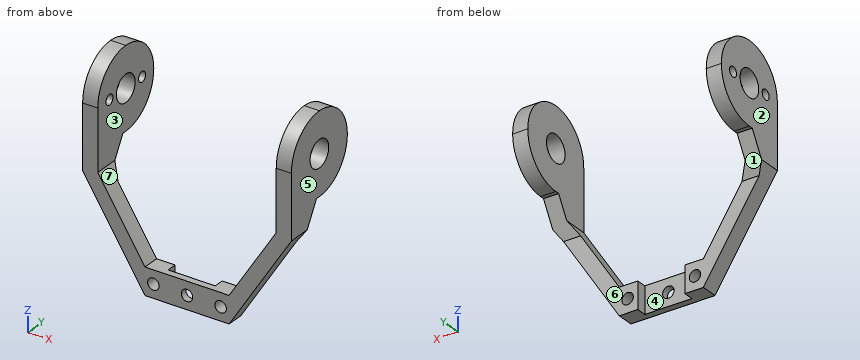
from build123d import *
from OCP.BRepFilletAPI import BRepFilletAPI_MakeChamfer

# Parameters (mm, degrees)
BOSS_EXTRUDE1_DEPTH     = 5
SKETCH2_W               = 4.5
SKETCH2_H               = 24
BOSS_EXTRUDE2_DEPTH     = 19
CUT_EXTRUDE1_REACH      = 59.853
SKETCH5_R               = 1.7
CUT_EXTRUDE2_REACH      = 73.673
SKETCH6_W               = 14
SKETCH6_H               = 3
CUT_EXTRUDE3_REACH      = 78.859
SKETCH7_R               = 1.5
CUT_EXTRUDE4_DEPTH      = 77.85863647
CUT_EXTRUDE4_DEPTH_BACK = 77.85863647
SKETCH8_R               = 4
FILLET1_R               = 12
CHAMFER2_SIZE           = 10
CHAMFER2_SIZE2          = 5.773502692
CUT_EXTRUDE5_REACH      = 59.853
SKETCH10_R              = 1.7


with BuildPart() as part:
    # Sketch1 → Boss-Extrude1 (new body)
    with BuildSketch(Plane(origin=(0, 0, 0), x_dir=(1, 0, 0), z_dir=(0, 1, 0))):
        Polygon((-31, 15.928571429), (-31, -15), (-26.5, -15), (-26.5, 15), (-12.5, 37), (12.5, 37), (26.5, 15), (26.5, -15), (31, -15), (31, 15.928571429), (12.5, 45), (-12.5, 45), align=None)
    extrude(amount=BOSS_EXTRUDE1_DEPTH)

    # Sketch2 → Boss-Extrude2 (add)
    with BuildSketch(Plane(origin=(0, 5, 0), x_dir=(1, 0, 0), z_dir=(0, 1, 0))):
        with Locations((-28.75, -3)):
            Rectangle(SKETCH2_W, SKETCH2_H)
        with Locations((28.75, -3)):
            Rectangle(SKETCH2_W, SKETCH2_H)
    extrude(amount=BOSS_EXTRUDE2_DEPTH)

    # Sketch5 → Cut-Extrude1 (cut, up to next)
    with BuildSketch(Plane(origin=(0, 5, 0), x_dir=(1, 0, 0), z_dir=(0, 1, 0)), mode=Mode.PRIVATE) as cut_extrude1_sk1:
        with Locations(Location((0, 41, 0), (0, 0, 270))):
            Circle(SKETCH5_R)
    cut_extrude1_tool1 = extrude(cut_extrude1_sk1.sketch, amount=-CUT_EXTRUDE1_REACH, mode=Mode.PRIVATE) & part.part
    add(cut_extrude1_tool1.solids().sort_by_distance((0, 5, -41))[0], mode=Mode.SUBTRACT)

    # Cut-Extrude2: up to this face of the body (flat: up to its plane)
    cut_extrude2_end = Plane(part.part.faces().sort_by_distance((0, 2.5, -37))[0])
    # Sketch6 → Cut-Extrude2 (cut, up to the picked face)
    with BuildSketch(Plane(origin=(0, 0, -45), x_dir=(-1, 0, 0), z_dir=(0, 0, -1)), mode=Mode.PRIVATE) as cut_extrude2_sk1:
        with Locations((0, 3.5)):
            Rectangle(SKETCH6_W, SKETCH6_H)
    cut_extrude2_tool1 = split(extrude(cut_extrude2_sk1.sketch, amount=-CUT_EXTRUDE2_REACH, mode=Mode.PRIVATE), bisect_by=cut_extrude2_end, keep=Keep.BOTH, mode=Mode.PRIVATE)
    add(cut_extrude2_tool1.solids().sort_by(Axis((0, 3.5, -45), (0, 0, 1)))[0], mode=Mode.SUBTRACT)

    # Sketch7 → Cut-Extrude3 (cut, up to next)
    with BuildSketch(Plane(origin=(-26.5, 0, 0), x_dir=(0, 0, -1), z_dir=(1, 0, 0)), mode=Mode.PRIVATE) as cut_extrude3_sk1:
        with Locations((-3, 19)):
            Circle(SKETCH7_R)
    cut_extrude3_tool1 = extrude(cut_extrude3_sk1.sketch, amount=-CUT_EXTRUDE3_REACH, mode=Mode.PRIVATE) & part.part
    # Sketch7 → Cut-Extrude3 (cut, up to next)
    with BuildSketch(Plane(origin=(-26.5, 0, 0), x_dir=(0, 0, -1), z_dir=(1, 0, 0)), mode=Mode.PRIVATE) as cut_extrude3_sk2:
        with Locations((-3, 5)):
            Circle(SKETCH7_R)
    cut_extrude3_tool2 = extrude(cut_extrude3_sk2.sketch, amount=-CUT_EXTRUDE3_REACH, mode=Mode.PRIVATE) & part.part
    add(cut_extrude3_tool1.solids().sort_by_distance((-26.5, 19, 3))[0], mode=Mode.SUBTRACT)
    add(cut_extrude3_tool2.solids().sort_by_distance((-26.5, 5, 3))[0], mode=Mode.SUBTRACT)

    # Sketch8 → Cut-Extrude4 (cut, two sides: drawn at the far end of the back side and taken through both)
    with BuildSketch(Plane(origin=(-26.5, 0, 0), x_dir=(0, 0, -1), z_dir=(1, 0, 0)).offset(-CUT_EXTRUDE4_DEPTH_BACK)):
        with Locations((-3, 12)):
            Circle(SKETCH8_R)
    extrude(amount=CUT_EXTRUDE4_DEPTH + CUT_EXTRUDE4_DEPTH_BACK, mode=Mode.SUBTRACT)

    # Fillet1
    fillet1_edges = [part.edges().sort_by_distance(p)[0] for p in [
        (28.75, 0, 15),
        (-28.75, 0, 15),
        (-28.75, 24, -9),
        (28.75, 24, -9),
        (28.75, 24, 15),
        (-28.75, 24, 15),
    ]]
    fillet(fillet1_edges, radius=FILLET1_R - 0.0001)  # a hair under: the kernel refuses the full size

    # Chamfer2: one chamfer whose edges measure the first distance from different faces: ONE call of the kernel's chamfer builder (chamfer() names one face for all edges)
    chamfer2_edges_1 = [part.edges().sort_by_distance(p)[0] for p in [
        (-28.75, 5, -9),
    ]]
    chamfer2_side_1 = [part.faces().sort_by_distance(p)[0] for p in [
        (-19.473621736, 5, -28.773341624),
    ]]
    chamfer2_edges_2 = [part.edges().sort_by_distance(p)[0] for p in [
        (28.75, 5, -9),
    ]]
    chamfer2_side_2 = [part.faces().sort_by_distance(p)[0] for p in [
        (19.473621736, 5, -28.773341624),
    ]]
    chamfer2 = BRepFilletAPI_MakeChamfer(part.part.solid().wrapped)
    for e in chamfer2_edges_1:
        chamfer2.Add(CHAMFER2_SIZE, CHAMFER2_SIZE2, e.wrapped, chamfer2_side_1[0].wrapped)  # the first distance lies on this face
    for e in chamfer2_edges_2:
        chamfer2.Add(CHAMFER2_SIZE, CHAMFER2_SIZE2, e.wrapped, chamfer2_side_2[0].wrapped)  # the first distance lies on this face
    add(Compound.cast(chamfer2.Shape()), mode=Mode.REPLACE)

    # Sketch10 → Cut-Extrude5 (cut, up to next)
    with BuildSketch(Plane(origin=(0, 5, 0), x_dir=(1, 0, 0), z_dir=(0, 1, 0)), mode=Mode.PRIVATE) as cut_extrude5_sk1:
        with Locations(Location((-10, 41, 0), (0, 0, 270))):
            Circle(SKETCH10_R)
    cut_extrude5_tool1 = extrude(cut_extrude5_sk1.sketch, amount=-CUT_EXTRUDE5_REACH, mode=Mode.PRIVATE) & part.part
    cut_extrude5 = cut_extrude5_tool1.solids().sort_by_distance((-10, 5, -41))[0]
    add(cut_extrude5, mode=Mode.SUBTRACT)

    # Mirror1: Cut-Extrude5 across plane
    add(cut_extrude5.mirror(Plane(origin=(0, 0, 0), x_dir=(0, 0, 1), z_dir=(1, 0, 0))), mode=Mode.SUBTRACT)


solid = part.part
Here's how the part is built. I have some questions about the finished solid (model axes, mm). Face numbers are marked on the shaded views. A direction names the side the tool comes from. Coordinates: 2 decimals unless noted, no trailing zeros. Order: outer loops, then holes, each group sorted by start corner. A loop starts at its lowest first (then second) coordinate and runs counter-clockwise, first axis right, second up.
Item 1: For P1, Ø5.5, axis at x = -10, z = -41, coming from the +Y side; P2, Ø12, axis at x = -18.5, z = 4.5, coming from the +Y side; P3, Ø1.5, axis at x = 3, y = 2.5, coming from the +Z side; P4, Ø0.9, axis at y = 4, z = -42.5, coming from the -X side, each with a flat end and sliding along its axis, tell me the tip position at first contact or that it passes through.
Result sheet:
P1: stops at y = 5
P2: passes through
P3: stops at z = -37
P4: stops at x = -14.38
Item 2: If we section it at C-C on y = 9.75: List the corners of the cut face in (x, z) for me, plus the area to 3 significant figures.
Result sheet:
outline: (-31, -10.77) - (-26.5, -10.77) - (-26.5, -0.31) - (-31, -0.31) - close; (-31, 6.31) - (-26.5, 6.31) - (-26.5, 14.79) - (-31, 14.79) - close; (26.5, -10.77) - (31, -10.77) - (31, -0.31) - (26.5, -0.31) - close; (26.5, 6.31) - (31, 6.31) - (31, 14.79) - (26.5, 14.79) - close
area: 171 mm2
Item 3: If we section it at A-A on x = 0: List the corners of the cut face in (y, z) for me, plus the area to 3 significant figures.
Result sheet:
outline: (0, -45) - (2, -45) - (2, -42.7) - (0, -42.7) - close; (0, -39.3) - (2, -39.3) - (2, -37) - (0, -37) - close
area: 9.20 mm2
Item 4: For the marked faces 5, 6 and 7, which set-ups out of +Z, -Z, +X, -X, +Y, -Y let a thin tool reach every point of the face, with its end or its side?
Result sheet:
face 5: +Z, -Z, +X, +Y, -Y
face 6: -Z, +X, -X, +Y
face 7: +Z, +Y, -Y
Item 5: I need wall thicknesses on line 1 (Y direction, x = -28.3, z = 3); line 2 (X direction, y = 13, z = -3.5); line 3 (X direction, y = 1.55, z = -41). Which ranges of each line are inside material? Lowest first, please.
Result sheet:
line 1: y = 0 to 3.5, 6.5 to 8, 16 to 17.5, 20.5 to 24
line 2: x = -31 to -26.5, 26.5 to 31
line 3: x = -15.05 to -11.7, -8.3 to -1.7, 1.7 to 8.3, 11.7 to 15.05
Item 6: If we section it at B-B on z = -35: List the corners of the cut face in (x, y) for me.
Result sheet:
outline: (-18.86, 0) - (-13.77, 0) - (-13.77, 5) - (-18.86, 5) - close; (13.77, 0) - (18.86, 0) - (18.86, 5) - (13.77, 5) - close
Item 7: If we section it at D-D on z = -41: List the corners of the cut face in (x, y) for me, plus the area to 3 significant figures.
Result sheet:
outline: (-15.05, 0) - (-11.7, 0) - (-11.7, 5) - (-15.05, 5) - close; (-8.3, 0) - (-1.7, 0) - (-1.7, 2) - (-7, 2) - (-7, 5) - (-8.3, 5) - close; (1.7, 0) - (8.3, 0) - (8.3, 5) - (7, 5) - (7, 2) - (1.7, 2) - close; (11.7, 0) - (15.05, 0) - (15.05, 5) - (11.7, 5) - close
area: 67.7 mm2
Item 8: If we mould it in two halves opening along X, with no side actions, what happens to the marked faces 1, 2, 3 and 4? For each: +X half, -X half, draft (parallel to the pull), parting line (faces both ways), or undercut.
Result sheet:
face 1: draft
face 2: -X half
face 3: undercut
face 4: undercut
